Here's the drawing with two shaded views (mm, measured from the low corner). I have some questions. A direction names the side the tool comes from. Round coordinates to 2 decimals unless told otherwise and drop trailing zeros. Order: outer loops, then holes, each group sorted by start corner. A loop starts at its lowest first (then second) coordinate and runs counter-clockwise, first axis right, second up. Notation, with made-up numbers: (29, 27) - (38, 27) arc R21 cw to (38, 41) - close; hole circle Ø2 at (-36, 80.5). An arc over 180 degrees is marked (long way). One line per item, written item: value.
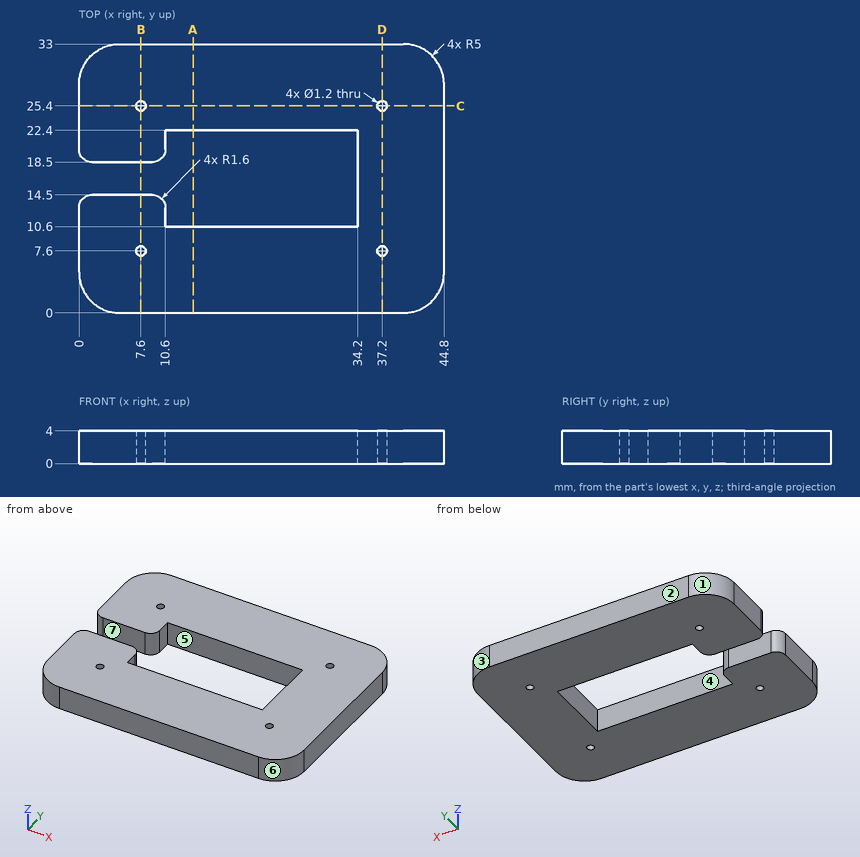
Q1. If we section it at B-B, the plane x = 7.6: Please give me the cut outline in (y, z), then the cut area to 3 significant figures.
Results list:
outline: (0, 0) - (7, 0) - (7, 4) - (0, 4) - close; (8.2, 0) - (14.5, 0) - (14.5, 4) - (8.2, 4) - close; (18.5, 0) - (24.8, 0) - (24.8, 4) - (18.5, 4) - close; (26, 0) - (33, 0) - (33, 4) - (26, 4) - close
area: 106 mm²
Q2. If I drill on line 1 along Y through (x, z) = (37.2, 2); line 2 along X through (y, z) = (25.5, 0.55); line 3 along Y through (x, z) = (18, 0.9), over which ranges is the centre line in solid material (lowest first)?
Results list:
line 1: 0 to 7, 8.2 to 24.8, 26 to 33
line 2: 0 to 7.01, 8.19 to 36.61, 37.79 to 44.8
line 3: 0 to 10.6, 22.4 to 33
Q3. We'd pull the mould along X, two halves only. Please class the marked faces 1, 2, 3 and 4: released by +X, released by -X, zero draft, split by the parting line, or undercut.
Results list:
face 1: released by -X
face 2: zero draft
face 3: released by +X
face 4: undercut
Q4. Which directions (+Z, -Z, +X, -X, +Y, -Y) give clear straight access to the entire face, cutting with the end or side of a thin tool? Please do the marked faces 5, 6 and 7.
Results list:
face 5: +Z, -Z
face 6: +Z, -Z, +X, -Y
face 7: +Z, -Z, -X
Q5. If we section it at D-D, the plane x = 37.2: Please give me the cut outline in (y, z).
Results list:
outline: (0, 0) - (7, 0) - (7, 4) - (0, 4) - close; (8.2, 0) - (24.8, 0) - (24.8, 4) - (8.2, 4) - close; (26, 0) - (33, 0) - (33, 4) - (26, 4) - close
Q6. If we section it at C-C, the plane y = 25.4: Please give me the cut outline in (x, z), then the cut area to 3 significant figures.
Results list:
outline: (0, 0) - (7, 0) - (7, 4) - (0, 4) - close; (8.2, 0) - (36.6, 0) - (36.6, 4) - (8.2, 4) - close; (37.8, 0) - (44.8, 0) - (44.8, 4) - (37.8, 4) - close
area: 170 mm²
Q7. If we section it at A-A, the plane x = 14: Please give me the cut outline in (y, z).
Results list:
outline: (0, 0) - (10.6, 0) - (10.6, 4) - (0, 4) - close; (22.4, 0) - (33, 0) - (33, 4) - (22.4, 4) - close
Q8. Will this pin go through, and if not, where does the flat tip stop? pin 1 (1 mm diameter, centred on x = 37.2, y = 7.6, fed in from +Z).
Results list:
pin 1: through
